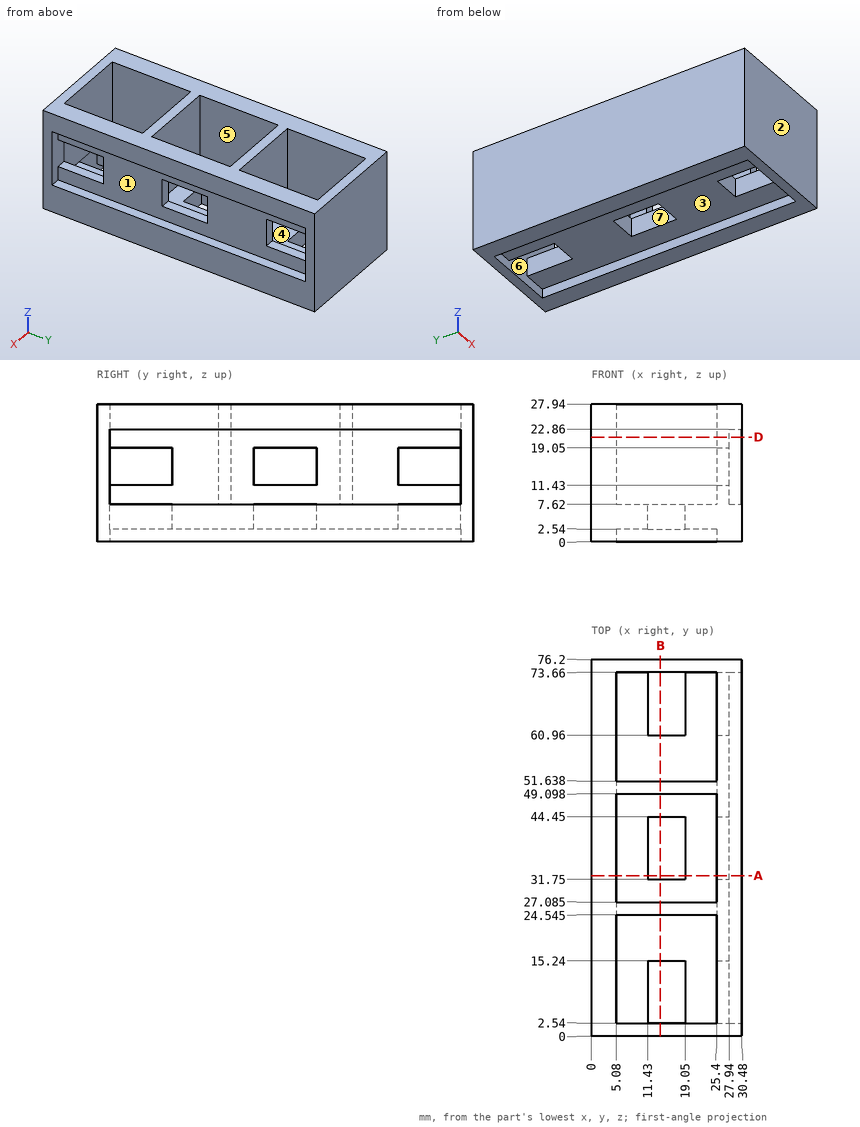
Input: dimensioned drawing with shaded views. Units: mm. Origin: part minimum x, y, z. A direction names the side the tool comes from. Coordinates: 2 decimals unless noted, no trailing zeros. Loops run counter-clockwise (first coordinate to the right, second up) from the corner with the lowest first, then second, coordinate; pieces in that order, holes last. Notation, with made-up numbers: (54.25, 86) - (86.25, 86) arc R15 ccw to (86.25, 115) - close; hole circle Ø2 at (69, 57.5). An arc over 180 degrees is marked (long way). One line per question, with ' | ' between items. Start each with the question number.
(1) Cut plane A-A on y = 32.5. Output: boundary loops of the cut face in (x, z), and give its area (3 significant figures).
(2) Draft query along Z for the marked faces 1, 2, 3 and 4. Return one class per face: +Z half, -Z half, draft (parallel to the pull), parting line (faces both ways), or undercut.
(3) Cut plane D-D on z = 21.25. Output: boundary loops of the cut face in (x, y) (1 decimal).
(4) Reachability of the marked faces 5, 6 and 7 from +Z, -Z, +X, -X, +Y, -Y: full face, straight path, thin tool, end or side. Return the list, or none.
(5) Ray query, L1, parallel to Y at x = 7.5, z = 10.5 (1 decimal); L2, parallel to X at y = 30, z = 19.75; L3, parallel to X at y = 56.5, z = 24.5. Return the intervals inside material, ascending. Write a range as from..to.
(6) First-contact query: pin 1 (16.5 mm diameter, centred on x = 14.5, y = 38.5, fed in from +Z); pin 2 (4 mm diameter, centred on x = 22.5, y = 35, fed in from -Z); pin 3 (6 mm diameter, centred on y = 43.5, z = 14, fed in from +X). Flat tips, straight axial feed; report the tip coordinate or a pass-through.
(7) Cut plane B-B on x = 14. Count the separate pieces of the cut face and the enclosed holes in it, and give its area (3 significant figures).
Here are the results:
1) outline: (0, 0) - (5.08, 0) - (5.08, 2.54) - (11.43, 2.54) - (11.43, 7.62) - (5.08, 7.62) - (5.08, 27.94) - (0, 27.94) - close; (19.05, 2.54) - (25.4, 2.54) - (25.4, 0) - (30.48, 0) - (30.48, 7.62) - (27.94, 7.62) - (27.94, 11.43) - (25.4, 11.43) - (25.4, 7.62) - (19.05, 7.62) - close; (25.4, 19.05) - (27.94, 19.05) - (27.94, 22.86) - (30.48, 22.86) - (30.48, 27.94) - (25.4, 27.94) - close | area: 290 mm²
2) face 1: undercut | face 2: draft | face 3: -Z half | face 4: +Z half
3) outline: (0, 0) - (30.5, 0) - (30.5, 2.5) - (27.9, 2.5) - (27.9, 73.7) - (30.5, 73.7) - (30.5, 76.2) - (0, 76.2) - close; hole (5.1, 2.5) - (25.4, 2.5) - (25.4, 24.5) - (5.1, 24.5) - close; hole (5.1, 27.1) - (25.4, 27.1) - (25.4, 49.1) - (5.1, 49.1) - close; hole (5.1, 51.6) - (25.4, 51.6) - (25.4, 73.7) - (5.1, 73.7) - close
4) face 5: +Z | face 6: none | face 7: +Z, -Z
5) L1: 0..2.5, 24.5..27.1, 49.1..51.6, 73.7..76.2 | L2: 0..5.08, 25.4..27.94 | L3: 0..5.08, 25.4..30.48
6) pin 1: z = 7.62 | pin 2: z = 2.54 | pin 3: x = 27.94
7) separate pieces: 4 | enclosed holes: 0 | area: 413 mm²
